Here's how the part is built. I have some questions about the finished solid (model axes, mm). A direction names the side the tool comes from. Round coordinates to 2 decimals unless told otherwise and drop trailing zeros. Order: outer loops, then holes, each group sorted by start corner. A loop starts at its lowest first (then second) coordinate and runs counter-clockwise, first axis right, second up. Notation, with made-up numbers: (73.5, -33) -> (82.5, -33) arc R16 cw to (82.5, -28) -> close; hole circle Ø3 at (72, -14). An arc over 180 degrees is marked (long way). Answer in a Markdown table with one row per item.
Autodesk Fusion 360 part; units mm, degrees
sketch "Sketch1" plane through (0, 0, 0) normal (0, 0, 1) x (1, 0, 0)
  line L0 (5.55, 9.3) -> (-5.55, 9.3)
  line L1 (-5.55, 9.3) -> (-5.55, -9.3)
  line L2 (-5.55, -9.3) -> (5.55, -9.3)
  line L3 (5.55, -9.3) -> (5.55, 9.3)
  line L4 (5.55, 9.3) -> (-5.55, -9.3) construction
  line L5 (-5.55, 9.3) -> (5.55, -9.3) construction
  line L6 (7.05, -10.8) -> (-7.05, -10.8)
  line L7 (-7.05, -10.8) -> (-7.05, 10.8)
  line L8 (-7.05, 10.8) -> (7.05, 10.8)
  line L9 (7.05, 10.8) -> (7.05, -10.8)
  line L10 (7.05, -10.8) -> (-7.05, 10.8) construction
  line L11 (-7.05, -10.8) -> (7.05, 10.8) construction
  line L12 (5.05, -8.8) -> (-5.05, -8.8)
  line L13 (-5.05, -8.8) -> (-5.05, 8.8)
  line L14 (-5.05, 8.8) -> (5.05, 8.8)
  line L15 (5.05, 8.8) -> (5.05, -8.8)
  line L16 (5.05, -8.8) -> (-5.05, 8.8) construction
  line L17 (-5.05, -8.8) -> (5.05, 8.8) construction
  dimension "d1" = 11.1
  dimension "d2" = 18.6
  dimension "d3" = 14.1
  dimension "d4" = 21.6
  dimension "d5" = 10.1
  dimension "d6" = 17.6
extrude "Extrude1" add sketch "Sketch1" along normal blind 1 contours L0 L1 L2 L3 | L6 L7 L8 L9
extrude "Extrude2" add sketch "Sketch1" against normal blind 3 contours L0 L1 L2 L3
sketch "Sketch2" plane through (0, 0, -3) normal (0, 0, -1) x (1, 0, 0)
  line L0 (5.05, -8.8) -> (-5.05, -8.8)
  line L1 (-5.05, -8.8) -> (-5.05, 8.8)
  line L2 (-5.05, 8.8) -> (5.05, 8.8)
  line L3 (5.05, 8.8) -> (5.05, -8.8)
  line L4 (5.55, -9.3) -> (5.55, 9.3)
  line L5 (5.55, 9.3) -> (-5.55, 9.3)
  line L6 (-5.55, 9.3) -> (-5.55, -9.3)
  line L7 (-5.55, -9.3) -> (5.55, -9.3)
  line L8 (5.55, -9.3) -> (-5.55, -9.3)
  line L9 (-5.55, -9.3) -> (-5.55, 9.3)
  line L10 (-5.55, 9.3) -> (5.55, 9.3)
  line L11 (5.55, 9.3) -> (5.55, -9.3)
  line L12 (5.55, -9.3) -> (-5.55, 9.3) construction
  line L13 (-5.55, -9.3) -> (5.55, 9.3) construction
  line L14 (4.35, -8.15) -> (-4.35, -8.15)
  line L15 (-4.35, -8.15) -> (-4.35, 8.15)
  line L16 (-4.35, 8.15) -> (4.35, 8.15)
  line L17 (4.35, 8.15) -> (4.35, -8.15)
  line L18 (4.35, -8.15) -> (-4.35, 8.15) construction
  line L19 (-4.35, -8.15) -> (4.35, 8.15) construction
  dimension "d11" = 8.7
  dimension "d12" = 16.3
extrude "Extrude3" add sketch "Sketch2" along normal blind 1 contours L0 L1 L2 L3 | L4 L5 L6 L7 L8 L9 L10 L11
fillet "Fillet1" radius 0.5 8 edges at (-7.05, -10.8, 0.5) (7.05, -10.8, 0.5) (-5.55, -9.3, -2) (5.55, -9.3, -2) (-5.55, 9.3, -2) (-7.05, 10.8, 0.5) (5.55, 9.3, -2) (7.05, 10.8, 0.5)
fillet "Fillet2" radius 0.5 8 edges at (6.9036, -10.6536, 1) (7.05, 0, 1) (6.9036, 10.6536, 1) (0, 10.8, 1) (-6.9036, 10.6536, 1) (-7.05, 0, 1) (-6.9036, -10.6536, 1) (0, -10.8, 1)
1. For pin 1 Ø3 at (y, z) = (4, -2.5) entering from -X; pin 2 Ø0.5 at (x, z) = (0, -3.5) entering from -Y; pin 3 Ø1.1 at (x, z) = (0.5, -3.5) entering from +Y, each with a flat end and sliding along its axis, tell me the tip position at first contact or that it passes through.
Numbers:
| item | result |
|---|---|
| pin 1 | stops at x = -5.55 |
| pin 2 | stops at y = -9.3 |
| pin 3 | stops at y = 9.3 |
2. Suppose I cut it at C-C on x = 2. Write out the boundary of the cut face in (y, z).
Numbers:
| item | result |
|---|---|
| outline | (-10.8, 0) -> (-9.3, 0) -> (-9.3, -4) -> (-8.15, -4) -> (-8.15, -3) -> (-8.8, -3) -> (-8.8, 1) -> (-10.3, 1) arc R0.5 ccw to (-10.8, 0.5) -> close; (8.15, -4) -> (9.3, -4) -> (9.3, 0) -> (10.8, 0) -> (10.8, 0.5) arc R0.5 ccw to (10.3, 1) -> (8.8, 1) -> (8.8, -3) -> (8.15, -3) -> close |
3. We'd pull the mould along Y, two halves only. Please class faces 1 (the face through (-5.55, 0, -2)), 2 (the face through (0, 9.3, -2)), 3 (the face through (0, -8.8, -1)): released by +Y, released by -Y, zero draft, split by the parting line, or undercut.
Numbers:
| item | result |
|---|---|
| face 1 | zero draft |
| face 2 | released by +Y |
| face 3 | undercut |
4. For faces 4 (the face through (0, -9.3, -2)), 5 (the face through (5.55, 0, -2)), 6 (the face through (-5.05, 0, -1)), 7 (the face through (-4.35, 0.1, -3.5)), which set-ups out of +Z, -Z, +X, -X, +Y, -Y let a thin tool reach every point of the face, with its end or its side?
Numbers:
| item | result |
|---|---|
| face 4 | -Z, +X, -X, -Y |
| face 5 | -Z, +X, +Y, -Y |
| face 6 | +Z |
| face 7 | +Z, -Z |
5. Suppose I cut it at B-B on z = -3.4. Write out the boundary of the cut face in (x, y).
Numbers:
| item | result |
|---|---|
| outline | (-5.55, -8.8) arc R0.5 ccw to (-5.05, -9.3) -> (5.05, -9.3) arc R0.5 ccw to (5.55, -8.8) -> (5.55, 8.8) arc R0.5 ccw to (5.05, 9.3) -> (-5.05, 9.3) arc R0.5 ccw to (-5.55, 8.8) -> close; hole (-4.35, -8.15) -> (4.35, -8.15) -> (4.35, 8.15) -> (-4.35, 8.15) -> close |
6. Please list where these lines run through material, in increasing order: line 1 along Y through (x, z) = (3.75, -2); line 2 along X through (y, z) = (7.25, -0.5); line 3 along Y through (x, z) = (-3, 0.4).
Numbers:
| item | result |
|---|---|
| line 1 | y = -9.3 to -8.8, 8.8 to 9.3 |
| line 2 | x = -5.55 to -5.05, 5.05 to 5.55 |
| line 3 | y = -10.8 to -8.8, 8.8 to 10.8 |
7. Suppose I cut it at A-A on y = 2.5. Write out the boundary of the cut face in (x, z), then the cut area to 3 significant figures.
Numbers:
| item | result |
|---|---|
| outline | (-7.05, 0) -> (-5.55, 0) -> (-5.55, -4) -> (-4.35, -4) -> (-4.35, -3) -> (-5.05, -3) -> (-5.05, 1) -> (-6.55, 1) arc R0.5 ccw to (-7.05, 0.5) -> close; (4.35, -4) -> (5.55, -4) -> (5.55, 0) -> (7.05, 0) -> (7.05, 0.5) arc R0.5 ccw to (6.55, 1) -> (5.05, 1) -> (5.05, -3) -> (4.35, -3) -> close |
| area | 9.29 mm2 |
